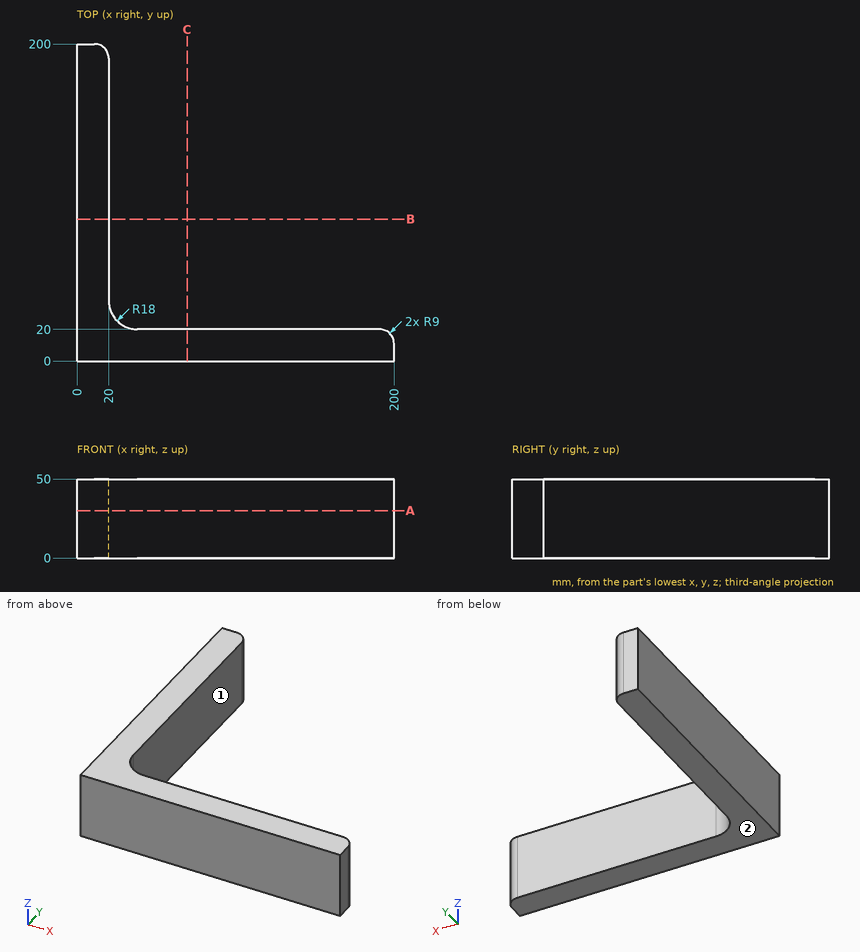
Source: three-view drawing plus pictorial views. Frame: mm from the lowest corner of the part. A direction names the side the tool comes from. Give positions to 0.01 mm unless a question says otherwise; leave off trailing zeros. Write each loop counter-clockwise with the first axis right and the second up, starting at its lowest first coordinate (ties: lowest second). Pieces come first, ordered by that corner, then holes. Notation, with made-up numbers: (36.25, 15.25) - (65.25, 15.25) arc R23 ccw to (65.25, 32.25) - close; hole circle Ø10 at (-20, 44.5). An arc over 180 degrees is marked (long way). Write item = value, one per line. Start each with the question number.
Q1. Material intervals for probe 1 along Y at (x, z) = (82.5, 36); probe 2 along Y at (x, z) = (26, 15.5), sorted ascending.
Q2. Reachability of the marked faces 1 and 2 from +Z, -Z, +X, -X, +Y, -Y: full face, straight path, thin tool, end or side. Return the list, or none.
Q3. Cut plane A-A, the plane z = 30. Return loops of the section in (x, y).
Q4. Pin query (flat end, axial travel): pin 1 Ø4 at (x, z) = (152, 29) entering from +Y; pin 2 Ø12 at (x, z) = (149, 28) entering from -Y; pin 3 Ø25 at (y, z) = (88, 22) entering from +X. Return the tip coordinate at first contact, or that it passes through.
Q5. Cut plane B-B, the plane y = 89.5. Return loops of the section in (x, z).
Computed values:
q1.probe_1 = 0 to 20
q1.probe_2 = 0 to 24.58
q2.face_1 = +Z, -Z, +X, +Y
q2.face_2 = -Z, +X, -X, +Y, -Y
q3.outline = (0, 0) - (200, 0) - (200, 11) arc R9 ccw to (191, 20) - (38, 20) arc R18 cw to (20, 38) - (20, 191) arc R9 ccw to (11, 200) - (0, 200) - close
q4.pin_1 = 20
q4.pin_2 = 0
q4.pin_3 = 20
q5.outline = (0, 0) - (20, 0) - (20, 50) - (0, 50) - close
